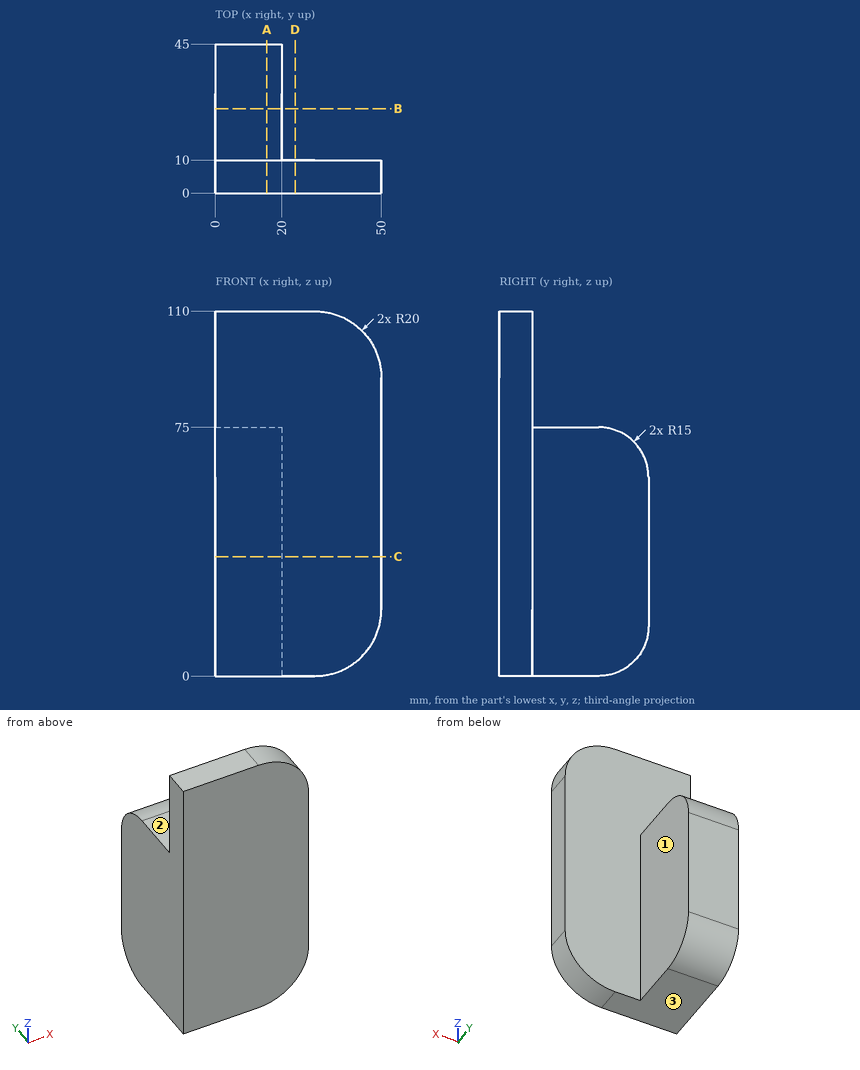
Study the drawing (mm; zero at the part's minimum x, y, z) and answer. A direction names the side the tool comes from. Give positions to 0.01 mm unless a question says otherwise; leave off trailing zeros. Write each loop counter-clockwise with the first axis right and the second up, starting at its lowest first coordinate (ties: lowest second). Pieces come first, ordered by that corner, then holes. Notation, with made-up numbers: (-9.75, -9) -> (46.25, -9) arc R20 ccw to (46.25, 11) -> close; hole circle Ø10 at (-37.5, -25). An arc over 180 degrees is marked (long way). Answer as a JSON object with one key per item and string values. Group by question number.
1) Find section D-D (x = 24). Write down the section's boundary in (y, z).
2) Each of these flat-tipped pins is pushed along its axis until it touches: P1, Ø15, axis at x = 31.5, z = 68, coming from the +Y side; P2, Ø8, axis at y = 30.5, z = 75.5, coming from the -X side; P3, Ø2, axis at y = 34, z = 33.5, coming from the +X side; P4, Ø4, axis at y = 38, z = 75.5, coming from the -X side. Where does it stop, or does it pass through?
3) Find section B-B (y = 25.5). Write down the section's boundary in (x, z), and give its area (3 significant figures).
4) Find section A-A (x = 15.5). Write down the section's boundary in (y, z), and give its area (3 significant figures).
5) Consider L1, parallel to X at y = 30.5, z = 6; L2, parallel to Y at x = 46.5, z = 61; L3, parallel to Z at x = 19, y = 19. Determine where each line is inside the solid, lowest interval first. Write a range as from..to.
6) A tool of negligible diameter and unlimited length cuts with its end or side. For the marked faces 1, 2 and 3, from which of +Z, -Z, +X, -X, +Y, -Y can it reach the whole face along a straight path? Write none if from no direction.
7) Find section C-C (z = 36). Write down the section's boundary in (x, y), and give its area (3 significant figures).
Values follow:
{
 "1": {"outline": "(0, 0) -> (10, 0) -> (10, 110) -> (0, 110) -> close"},
 "2": {"P1": "stops at y = 10", "P2": "stops at x = 0", "P3": "stops at x = 20", "P4": "passes through"},
 "3": {"outline": "(0, 0) -> (20, 0) -> (20, 75) -> (0, 75) -> close", "area": "1,500 mm2"},
 "4": {"outline": "(0, 0) -> (30, 0) arc R15 ccw to (45, 15) -> (45, 60) arc R15 ccw to (30, 75) -> (10, 75) -> (10, 110) -> (0, 110) -> close", "area": "3,630 mm2"},
 "5": {"L1": "x = 0..20", "L2": "y = 0..10", "L3": "z = 0..75"},
 "6": {"face 1": "+Z, -Z, +X, +Y", "face 2": "+Z, +X, -X, +Y", "face 3": "-Z, +X, -X, +Y, -Y"},
 "7": {"outline": "(0, 0) -> (50, 0) -> (50, 10) -> (20, 10) -> (20, 45) -> (0, 45) -> close", "area": "1,200 mm2"}
}
